Geometry: final body of the model. Coordinates: model frame, mm. A direction names the side the tool comes from. Give positions to 0.01 mm unless a question says otherwise; leave off trailing zeros. Write each loop counter-clockwise with the first axis right and the second up, starting at its lowest first coordinate (ties: lowest second). Pieces come first, ordered by that corner, then holes. Notation, with made-up numbers: (34, 12) - (80, 12) arc R25 ccw to (80, 24) - close; hole circle Ø10 at (-26.5, -15). An arc over 180 degrees is marked (long way). Use CSV: the item, a comma, the result in double quotes. Start each with the question number.
(1) Section B-B on z = 0. Output: boundary loops of the cut face in (x, y).
(2) Section C-C on x = 5. Output: boundary loops of the cut face in (y, z).
(3) Section D-D on y = -7.5. Output: boundary loops of the cut face in (x, z).
(4) Line query: probe 1 along Z at (x, y) = (5, 7.25); probe 2 along Y at (x, z) = (-2.75, 7.25). Output: solid intervals per line, ascending. Write a range as [from, to].
(5) Section A-A on y = 5.25. Output: boundary loops of the cut face in (x, z).
(6) First-contact query: pin 1 Ø1.5 at (y, z) = (6, 6) entering from -X; pin 2 Ø1 at (x, y) = (-0.5, -4) entering from -Z; pin 3 Ø10 at (y, z) = (-7, -4) entering from +X; pin 4 Ø1.4 at (x, z) = (5, 5) entering from -Y. Flat tips, straight axial feed; report the tip coordinate or a pass-through.
(7) Reachability of faces 5 (the cylindrical face through (-2.799, -4.93, -2.815)), 6 (the cylindrical face through (2.815, -4.93, -2.799)), 7 (the cylindrical face through (2.799, -4.93, 2.815)) from +Z, -Z, +X, -X, +Y, -Y: full face, straight path, thin tool, end or side. Return the list, or none.
(8) Draft query along Z for faces 1 (the cylindrical face through (5.63, 4.93, 5.49)), 2 (the cylindrical face through (-2.815, -4.93, 2.799)), 3 (the cylindrical face through (5.8, 4.9, -5)), 4 (the flat face through (0, 0, 4)). Return one class per face: released by +Z, released by -Z, zero draft, split by the parting line, or undercut.
from build123d import *

# Parameters (mm, degrees)
SKETCH1_R             = 10
BOSS_EXTRUDE1_DEPTH   = 10
M2X0_4_TAPPED_HOLE1_D = 1.6
BOSS_EXTRUDE2_DEPTH   = 10


with BuildPart() as part:
    # Sketch1 → Boss-Extrude1 (new body)
    with BuildSketch(Plane(origin=(0, 0, 0), x_dir=(1, 0, 0), z_dir=(0, 1, 0))):
        with Locations(Location((0, 0, 0), (0, 0, 270))):
            Circle(SKETCH1_R)
    extrude(amount=BOSS_EXTRUDE1_DEPTH)

    # M2x0.4 Tapped Hole1 (through all)
    with Locations(Plane(origin=(0, 10, 0), x_dir=(1, 0, 0), z_dir=(0, 1, 0))):
        with Locations((-5, 5), (5, 5), (5, -5), (-5, -5)):
            Hole(M2X0_4_TAPPED_HOLE1_D / 2)

    # Sketch5 → Boss-Extrude2 (add)
    with BuildSketch(Plane.XZ):
        with BuildLine():
            Line((-2.1, 3.1), (2.1, 3.1))
            ThreePointArc((2.1, 3.1), (2.807106781, 2.807106781), (3.1, 2.1))
            Line((3.1, 2.1), (3.1, -2.1))
            ThreePointArc((3.1, -2.1), (2.807106781, -2.807106781), (2.1, -3.1))
            Line((2.1, -3.1), (-2.1, -3.1))
            ThreePointArc((-2.1, -3.1), (-2.807106781, -2.807106781), (-3.1, -2.1))
            Line((-3.1, -2.1), (-3.1, 2.1))
            ThreePointArc((-3.1, 2.1), (-2.807106781, 2.807106781), (-2.1, 3.1))
        make_face()
    extrude(amount=BOSS_EXTRUDE2_DEPTH)


solid = part.part
Check values:
1,outline,"(-10, 0) - (-3.1, 0) - (-3.1, -10) - (3.1, -10) - (3.1, 0) - (10, 0) - (10, 10) - (-10, 10) - close"
2,outline,"(0, -8.66) - (10, -8.66) - (10, -5.8) - (0, -5.8) - close; (0, -4.2) - (10, -4.2) - (10, 4.2) - (0, 4.2) - close; (0, 5.8) - (10, 5.8) - (10, 8.66) - (0, 8.66) - close"
3,outline,"(-3.1, -2.1) arc R1 ccw to (-2.1, -3.1) - (2.1, -3.1) arc R1 ccw to (3.1, -2.1) - (3.1, 2.1) arc R1 ccw to (2.1, 3.1) - (-2.1, 3.1) arc R1 ccw to (-3.1, 2.1) - close"
4,probe 1,"z = [-8.66, -5.8], [-4.2, 4.2], [5.8, 8.66]"
4,probe 2,"y = [0, 10]"
5,outline,"circle Ø20 at (0, 0); hole circle Ø1.6 at (-5, -5); hole circle Ø1.6 at (-5, 5); hole circle Ø1.6 at (5, -5); hole circle Ø1.6 at (5, 5)"
6,pin 1,"stops at x = -8.51"
6,pin 2,"stops at z = -3.1"
6,pin 3,"stops at x = 3.1"
6,pin 4,"passes through"
7,face 5,"-Z, -X, -Y"
7,face 6,"-Z, +X, -Y"
7,face 7,"+Z, +X, -Y"
8,face 1,"undercut"
8,face 2,"released by +Z"
8,face 3,"undercut"
8,face 4,"zero draft"
